The model under review builds one solid part; all positions refer to its coordinate system, in mm. A direction names the side the tool comes from. Coordinates: 2 decimals unless noted, no trailing zeros. Write each loop counter-clockwise with the first axis right and the second up, starting at its lowest first coordinate (ties: lowest second). Pieces come first, ordered by that corner, then holes. Notation, with made-up numbers: M 5.25,25.5 L 33.25,25.5 A20 cw 33.25,29.5 Z; hole C 60.25,68.5 d7. An arc over 180 degrees is marked long. Answer as a JSON object with one key per item and string values.
```python
from build123d import *

# Parameters (mm, degrees)
F1_DEPTH  = 4
F2_W      = 4
F2_H      = 16
F2_W_2    = 20
F2_H_2    = 4
F3_DEPTH  = 24
F5_DEPTH  = 20
F7_DEPTH  = 20
F8_SIZE   = 10
F9_SIZE   = 5
F10_R     = 2
F10_R_2   = 2.1593554105
F11_DEPTH = 20.1
F13_DEPTH = 3.5
F15_DEPTH = 3.5


with BuildPart() as f1:
    # F0 (on Top) → F1 (new body)
    with BuildSketch(Plane.XY):
        Polygon((-35.7348556412, 8.7559268959), (-77.3040750229, 8.7559268959), (-77.3040750229, -15.2440731041), (-29.3040750229, -15.2440731041), (-29.3040750229, -2.3825118674), align=None)
        Polygon((90.6959249771, 81.7507721197), (-35.7348556412, 8.7559268959), (-29.3040750229, 8.7559268959), (-29.3040750229, -2.3825118674), (-23.7348556412, -12.0286827949), (102.6959249771, 60.9661624289), align=None)
        Polygon((-29.3040750229, 8.7559268959), (-35.7348556412, 8.7559268959), (-29.3040750229, -2.3825118674), align=None)
        Polygon((-23.7348556412, -12.0286827949), (-29.3040750229, -2.3825118674), (-29.3040750229, -15.2440731041), align=None)
    extrude(amount=F1_DEPTH)

    # F2 (on face) → F3 (join)
    with BuildSketch(Plane.XZ.offset(15.2440731041)):
        with Locations((-31.3040750229, 12)):
            Rectangle(F2_W, F2_H)
        Polygon((-33.3040750229, 20), (-29.3040750229, 20), (-29.3040750229, 24), (-33.1334466886, 24), (-57.3040750229, 23), (-57.3040750229, 19), align=None)
        with Locations((-67.3040750229, 21)):
            Rectangle(F2_W_2, F2_H_2)
    extrude(amount=-F3_DEPTH)

    # F4 (on face) → F5 (join)
    with BuildSketch(Plane.XY.offset(4)):
        Polygon((-29.3040750229, -3.6970677203), (97.6959249771, 69.6264164668), (95.6959249771, 73.0905180819), (-29.3040750229, 0.9217344332), align=None)
    extrude(amount=F5_DEPTH)

    # F6 (on face) → F7 (join)
    with BuildSketch(Plane.XY.offset(4)):
        Polygon((87.0356709393, 68.0905180819), (95.6959249771, 73.0905180819), (90.6959249771, 81.7507721197), (82.0356709393, 76.7507721197), align=None)
        Polygon((4.7632575798, 20.5905180819), (-0.2367424202, 29.2507721197), (-8.8969964581, 24.2507721197), (-3.8969964581, 15.5905180819), align=None)
    extrude(amount=F7_DEPTH)

    # F8
    f8_edges = [f1.edges().sort_by_distance(p)[0] for p in [
        (86.365798, 79.250772, 24),
        (-4.566869, 26.750772, 24),
    ]]
    chamfer(f8_edges, length=F8_SIZE)

    # F9
    f9_edges = [f1.edges().sort_by_distance(p)[0] for p in [
        (34.195925, 32.964674, 4),
        (45.899464, 44.340518, 4),
    ]]
    chamfer(f9_edges, length=F9_SIZE)

    # F10 (on face) → F11 (cut)
    with BuildSketch(Plane(origin=(-9.8625707365, 17.0824736089, 19.7251414731), x_dir=(0.9354143467, 0.2314550249, 0.2672612419), z_dir=(-0.3535533906, 0.6123724357, 0.7071067812))):
        with Locations((7.5511651872, 6.4274310849)):
            Circle(F10_R)
        with Locations((104.822506347, 45.9661663088)):
            Circle(F10_R_2)
    extrude(amount=-F11_DEPTH, mode=Mode.SUBTRACT)

    # F12 (on face) → F13 (cut)
    with BuildSketch(Plane(origin=(-9.8625707365, 17.0824736089, 19.7251414731), x_dir=(0.9354143467, 0.2314550249, 0.2672612419), z_dir=(-0.3535533906, 0.6123724357, 0.7071067812))):
        Polygon((101.187753457, 44.4822846552), (104.2902091103, 42.0764371428), (107.9249620003, 43.5603187964), (108.457259237, 47.4500479624), (105.3548035838, 49.8558954748), (101.7200506938, 48.3720138212), align=None)
    extrude(amount=-F13_DEPTH, mode=Mode.SUBTRACT)

    # F14 (on face) → F15 (cut)
    with BuildSketch(Plane(origin=(-9.8625707365, 17.0824736089, 19.7251414731), x_dir=(0.9354143467, 0.2314550249, 0.2672612419), z_dir=(-0.3535533906, 0.6123724357, 0.7071067812))):
        Polygon((3.9164122972, 4.9435494313), (7.0188679504, 2.5377019189), (10.6536208404, 4.0215835725), (11.1859180772, 7.9113127385), (8.0834624239, 10.3171602509), (4.4487095339, 8.8332785973), align=None)
    extrude(amount=-F15_DEPTH, mode=Mode.SUBTRACT)


solid = f1.part
```
(1) Add section B-B on y = 35. Give the boundary of the cut face in (x, z).
Results list:
{"outline": "M 9.72,0 L 57.72,0 L 57.72,4 L 47.72,4 L 37.72,9 L 37.72,24 L 29.72,24 L 29.72,9 L 19.72,4 L 9.72,4 Z"}
(2) Draft analysis for pull direction Y (two halves, no side actions). For faces 6 (the face through (4.28, 11.46, 3.24)), 7 (the face through (2.3, 24.86, 11.64)), 8 (the face through (36, 25, 4)), state which applies: released by +Y, released by -Y, zero draft, split by the parting line, or undercut.
Results list:
{"face 6": "undercut", "face 7": "released by +Y", "face 8": "zero draft"}
(3) Add section A-A on x = -37.5. Give the boundary of the cut face in (y, z).
Results list:
{"outline": "M -15.24,0 L 8.76,0 L 8.76,4 L -15.24,4 Z; M -15.24,19.83 L 8.76,19.83 L 8.76,23.82 L -15.24,23.82 Z"}
(4) For faces 1 (the face through (0.96, 23.04, 17.53)), 2 (the face through (-56, 8.756, 2)), 3 (the face through (-50, 8.756, 20)), 4 (the face through (-16.42, 8.36, 13.86)), 5 (the face through (84.5, 72.48, 11.64)), list the 3-axis set-ups (+Z, -Z, +X, -X, +Y, -Y) from which the entire face can be reached by the end or side of a thin tool; tool diameter is ignored.
Results list:
{"face 1": "none", "face 2": "+Z, -Z, -X, +Y", "face 3": "+Z, -X, +Y", "face 4": "+Z", "face 5": "+Z, -X"}
(5) For pin 1 Ø8 at (y, z) = (43.5, 16) entering from -X; pin 2 Ø22 at (x, y) = (-68.5, -1) entering from -Z; pin 3 Ø3.5 at (y, z) = (-10.5, 18.5) entering from +X; pin 4 Ø10 at (x, z) = (69, 21) entering from +Y, all flat-tipped, find the tip position at first contact; note any pin that passes through.
Results list:
{"pin 1": "x = 37.52", "pin 2": "z = 0", "pin 3": "x = -29.3", "pin 4": "y = 60.56"}
(6) Add section D-D on z = 11. Count the separate pieces of the cut face and the enclosed holes in it, and give its area (3 significant figures).
Results list:
{"separate pieces": "1", "enclosed holes": "2", "area": "839 mm²"}
(7) Add section C-C on x = 80. Give the boundary of the cut face in (y, z), and give its area (3 significant figures).
Results list:
{"outline": "M 47.86,0 L 75.58,0 L 75.58,4 L 69.8,4 L 64.03,9 L 64.03,24 L 59.41,24 L 59.41,9 L 53.64,4 L 47.86,4 Z", "area": "232 mm²"}
(8) Wall thickness on line 1 along X through (y, z) = (-8.5, 14); line 2 along Y through (x, z) = (-65, 20.75); line 3 along Z through (x, y) = (2.5, 17): over which ranges is each line inside the solid? List them lowest first. Write a range as from..to.
Results list:
{"line 1": "-33.3..-29.3", "line 2": "-15.24..8.76", "line 3": "0..6.88, 11.31..24"}
